Work out the finished part from the listing and answer in its coordinate system (mm). Round coordinates to 2 decimals unless told otherwise and drop trailing zeros. Order: outer loops, then holes, each group sorted by start corner. A loop starts at its lowest first (then second) coordinate and runs counter-clockwise, first axis right, second up. Notation, with made-up numbers: (67.25, 37) - (96.25, 37) arc R27 cw to (96.25, 70) - close; hole circle Ø7 at (2, -35). An arc over 180 degrees is marked (long way). Use CSV: the item, a comma, the result in double quotes.
from build123d import *

# Parameters (mm, degrees)
F1_DEPTH = 3.75


with BuildPart() as f1:
    # F0 (on Right) → F1 (new body, symmetric)
    with BuildSketch(Plane.YZ):
        Polygon((7.5, -203.2), (7.5, 203.2), (-7.5, 203.2), (-7.5, 188.2), (0, 188.2), (0, 180.7), (-7.5, 180.7), (-7.5, -180.7), (0, -180.7), (0, -188.2), (-7.5, -188.2), (-7.5, -203.2), align=None)
    extrude(amount=F1_DEPTH, both=True)


solid = f1.part
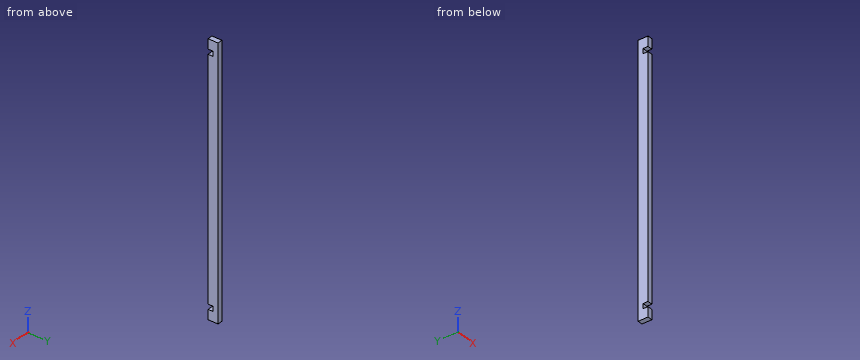
(1) Find section A-A (y = -3). Determine the outline of the cut face in (x, z), and give its area (3 significant figures).
Findings below:
outline,"(-3.75, -203.2) - (3.75, -203.2) - (3.75, -188.2) - (-3.75, -188.2) - close; (-3.75, -180.7) - (3.75, -180.7) - (3.75, 180.7) - (-3.75, 180.7) - close; (-3.75, 188.2) - (3.75, 188.2) - (3.75, 203.2) - (-3.75, 203.2) - close"
area,"2,940 mm²"
(2) Find section B-B (x = -1.25). Determine the outline of the cut face in (y, z), and give its area (3 significant figures).
Findings below:
outline,"(-7.5, -203.2) - (7.5, -203.2) - (7.5, 203.2) - (-7.5, 203.2) - (-7.5, 188.2) - (0, 188.2) - (0, 180.7) - (-7.5, 180.7) - (-7.5, -180.7) - (0, -180.7) - (0, -188.2) - (-7.5, -188.2) - close"
area,"5,980 mm²"
(3) Find the intervals of material crossed by L1, parallel to Z at x = 2.75, y = -2.75, in increasing order. Write a range as from..to.
Findings below:
L1,"z = -203.2..-188.2, -180.7..180.7, 188.2..203.2"
(4) This flat-tipped pin is pushed along its axis until it touches: pin 1 (4 mm diameter, centred on x = 0.5, z = 186, fed in from -Y). Where does it stop, or does it pass through?
Findings below:
pin 1,"stops at y = 0"
